Part model, mm, in its own coordinate system. A direction names the side the tool comes from. Coordinates: 2 decimals unless noted, no trailing zeros. Loops run counter-clockwise (first coordinate to the right, second up) from the corner with the lowest first, then second, coordinate; pieces in that order, holes last. Notation, with made-up numbers: M -39.75,7.5 L -33.75,7.5 A29 ccw -33.75,29.5 Z; hole C 22,31 d5. An arc over 180 degrees is marked long. Answer as a JSON object with one key per item and string values. Group by question number.
1. Drop flat-ended pins along their axis: pin 1 Ø10 at (y, z) = (9, 6) entering from +X; pin 2 Ø1.5 at (y, z) = (10.5, -12.5) entering from -X; pin 3 Ø7.5 at (x, z) = (-1.5, 0.5) entering from +Y. Give the stop position or say it passes through.
2. Saw through at B-B on x = -1.5. Write the cut outline in (y, z) (3 decimals), then the cut area to 3 significant figures.
3. Drill centre lines: L1, parallel to Y at x = 1.5, z = -4; L2, parallel to Z at x = -1.5, y = 3; L3, parallel to Z at x = 3, y = 9. Where is each one in solid material? Low to high.
4. Saw through at A-A on z = 0. Write the cut outline in (x, y).
5. Saw through at D-D on x = -4.75. Write the cut outline in (y, z).
6. Saw through at C-C on x = 4.5. Write the cut outline in (y, z), then the cut area to 3 significant figures.
7. Mould opens along Z. For faces 1 (the face through (0, 1, 2.515)), 2 (the face through (-2.17, 5.24, -9.97)), 3 (the face through (-3.49, 5.45, 16.07)) say: released by +Z, released by -Z, zero draft, split by the parting line, or undercut.
8. 3-axis set-ups, long thin cutter, end or side, ignore diameter. For faces 4 (the face through (0, 1, -2.515)), 5 (the face through (-3.49, 6.55, 15.77)), 6 (the face through (3.28, 7.928, -11.684)): which of +Z, -Z, +X, -X, +Y, -Y reach the whole face in a straight line?
from build123d import *

# Parameters (mm, degrees)
SKETCH1_W           = 15.24
SKETCH1_H           = 15.24
BOSS_EXTRUDE1_DEPTH = 1.2954
BOSS_EXTRUDE2_DEPTH = 15.24
CUT_EXTRUDE1_DEPTH  = 15.24
CUT_EXTRUDE2_DEPTH  = 15.24


with BuildPart() as part:
    # Sketch1 → Boss-Extrude1 (new body)
    with BuildSketch(Plane(origin=(0, 0, 0), x_dir=(1, 0, 0), z_dir=(0, 1, 0))):
        Rectangle(SKETCH1_W, SKETCH1_H)
        with BuildLine():
            Line((-0.43942, 2.5146), (0.43942, 2.5146))
            ThreePointArc((0.43942, 2.5146), (2.95402, 0), (0.43942, -2.5146))
            Line((0.43942, -2.5146), (-0.43942, -2.5146))
            ThreePointArc((-0.43942, -2.5146), (-2.95402, 0), (-0.43942, 2.5146))
        make_face(mode=Mode.SUBTRACT)
    extrude(amount=BOSS_EXTRUDE1_DEPTH)

    # Sketch3 → Boss-Extrude2 (add)
    with BuildSketch(Plane.ZY.offset(7.62)):
        Polygon((7.62, 1.2954), (28.967378653, 15.059462796), (28.967378653, 13.764062796), (7.62, 0), align=None)
        Polygon((-7.62, 1.2954), (-17.885578899, 21.321091109), (-17.885578899, 20.025691109), (-7.62, 0), align=None)
    extrude(amount=-BOSS_EXTRUDE2_DEPTH)

    # Sketch4 → Cut-Extrude1 (cut)
    with BuildSketch(Plane(origin=(0, -2.555384203, 1.647624714), x_dir=(1, 0, 0), z_dir=(0, 0.840447978, -0.541892236))):
        with BuildLine():
            Line((7.62, -7.106180798), (7.62, -32.506180798))
            Line((7.62, -32.506180798), (-7.62, -32.506180798))
            ThreePointArc((-7.62, -32.506180798), (-1.894391171, -27.153773172), (0, -19.548370753))
            ThreePointArc((0, -19.548370753), (2.118358532, -12.291259766), (7.62, -7.106180798))
        make_face()
    extrude(amount=-CUT_EXTRUDE1_DEPTH, mode=Mode.SUBTRACT)

    # Sketch5 → Cut-Extrude2 (cut)
    with BuildSketch(Plane(origin=(0, -2.823741084, -5.508444021), x_dir=(1, 0, 0), z_dir=(0, 0.456175683, 0.889889738))):
        with BuildLine():
            Line((-7.62, 4.628821871), (-7.62, 27.132386357))
            Line((-7.62, 27.132386357), (7.62, 27.132386357))
            ThreePointArc((7.62, 27.132386357), (2.681671235, 22.223683301), (0, 15.797868484))
            ThreePointArc((0, 15.797868484), (-2.22452861, 9.131668969), (-7.62, 4.628821871))
        make_face()
    extrude(amount=-CUT_EXTRUDE2_DEPTH, mode=Mode.SUBTRACT)


solid = part.part
Outcome:
{
 "1": {"pin 1": "passes through", "pin 2": "stops at x = -0.16", "pin 3": "stops at y = 1.3"},
 "2": {"outline": "M 0,-7.62 L 6.098,-10.746 L 6.368,-10.22 L 1.295,-7.62 L 1.295,-2.28 L 0,-2.28 Z; M 0,2.28 L 1.295,2.28 L 1.295,7.62 L 11.77,23.865 L 10.855,24.455 L 0,7.62 Z", "area": "39.0 mm²"},
 "3": {"L1": "y = 0 to 1.3", "L2": "z = -9.16 to -8.49, 10.26 to 12.27", "L3": "z = -12.23 to -11.57"},
 "4": {"outline": "M -7.62,0 L -2.95,0 L -2.95,1.3 L -7.62,1.3 Z; M 2.95,0 L 7.62,0 L 7.62,1.3 L 2.95,1.3 Z"},
 "5": {"outline": "M 0,-7.62 L 2.59,-8.95 L 2.86,-8.42 L 1.3,-7.62 L 1.3,7.62 L 14.02,27.35 L 13.1,27.94 L 0,7.62 Z"},
 "6": {"outline": "M 0,-7.62 L 18.71,-17.21 L 18.98,-16.69 L 1.3,-7.62 L 1.3,7.62 L 2.51,9.51 L 1.6,10.1 L 0,7.62 Z", "area": "34.7 mm²"},
 "7": {"face 1": "undercut", "face 2": "released by -Z", "face 3": "released by +Z"},
 "8": {"face 4": "+Y, -Y", "face 5": "+X, -X, +Y", "face 6": "-Z, +X, -X, -Y"}
}
